Geometry check sheet. Reference: drawing and pictorial views, mm from the part's lowest x, y, z. Round coordinates to 2 decimals unless told otherwise and drop trailing zeros. Write each loop counter-clockwise with the first axis right and the second up, starting at its lowest first coordinate (ties: lowest second). Pieces come first, ordered by that corner, then holes.
Item 1: Section check B-B, the plane z = 45. Record the cut outline in (x, y).
Item 2: Section check A-A, the plane x = 48. Record the cut outline in (y, z).
Item 3: Depth check by flat-ended pin: pin 1 (3 mm diameter, centred on y = 4, z = 40.5, fed in from -X); pin 2 (3 mm diameter, centred on x = 3, z = 3, fed in from +Y). Enter the tip coordinate at first touch or a pass-through.
Item 4: Material ranges on line 1 along X through (y, z) = (4.5, 3); line 2 along Z through (x, y) = (3, 2); line 3 along Z through (x, y) = (49, 6), recorded low to high.
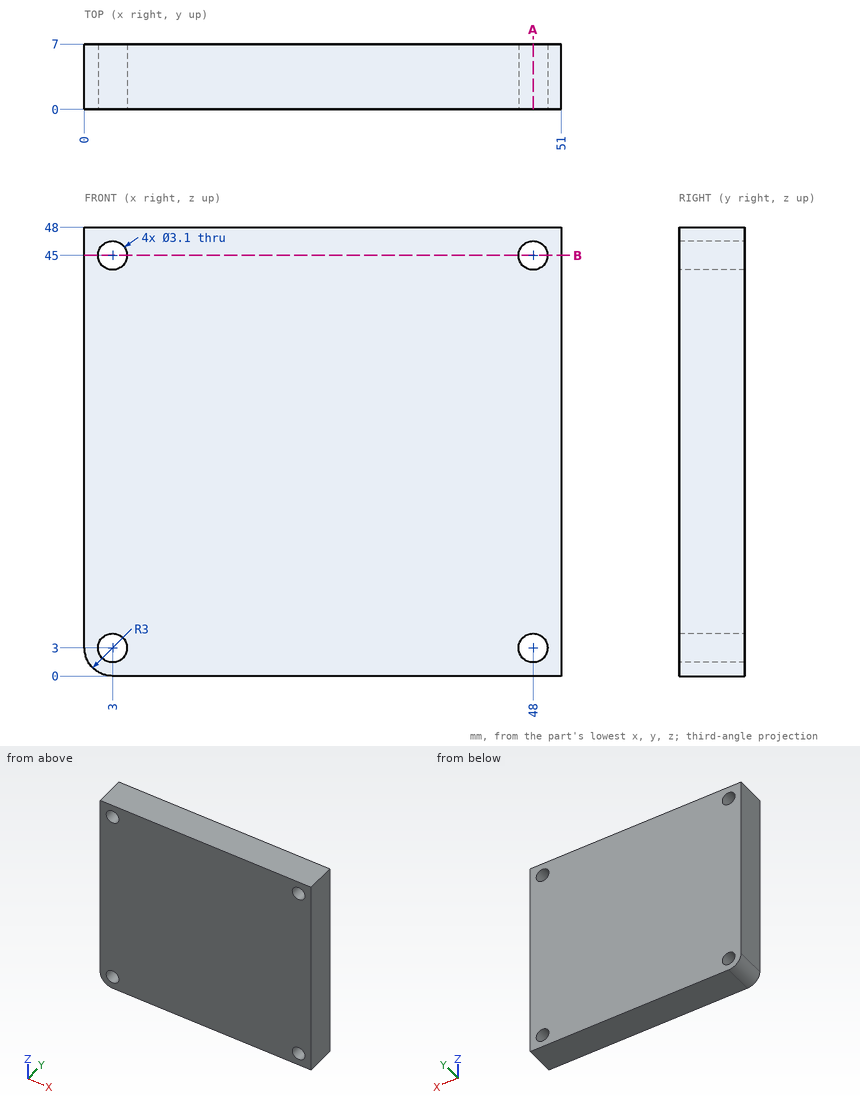
Values found:
1. outline: (0, 0) - (1.45, 0) - (1.45, 7) - (0, 7) - close; (4.55, 0) - (46.45, 0) - (46.45, 7) - (4.55, 7) - close; (49.55, 0) - (51, 0) - (51, 7) - (49.55, 7) - close
2. outline: (0, 0) - (7, 0) - (7, 1.45) - (0, 1.45) - close; (0, 4.55) - (7, 4.55) - (7, 43.45) - (0, 43.45) - close; (0, 46.55) - (7, 46.55) - (7, 48) - (0, 48) - close
3. pin 1: stops at x = 0
3. pin 2: passes through
4. line 1: x = 0 to 1.45, 4.55 to 46.45, 49.55 to 51
4. line 2: z = 0 to 1.45, 4.55 to 43.45, 46.55 to 48
4. line 3: z = 0 to 1.82, 4.18 to 43.82, 46.18 to 48
